Geometry: final body of the model. Coordinates: model frame, mm. Face numbers are marked on the shaded views. A direction names the side the tool comes from. Coordinates: 2 decimals unless noted, no trailing zeros. Loops run counter-clockwise (first coordinate to the right, second up) from the corner with the lowest first, then second, coordinate; pieces in that order, holes last. Notation, with made-up numbers: (17.25, 1) -> (63.25, 1) arc R15 ccw to (63.25, 6) -> close; hole circle Ø1 at (65.25, 55.25). An arc over 180 degrees is marked (long way). One line per item, written item: value. Start each with the question number.
Autodesk Inventor part; units mm, degrees
ref_plane "YZ Plane" through (0, 0, 0) normal (1, 0, 0) x (0, 1, 0)
ref_plane "XZ Plane" through (0, 0, 0) normal (0, 1, 0) x (-1, 0, 0)
ref_plane "XY Plane" through (0, 0, 0) normal (0, 0, 1) x (1, 0, 0)
sketch "Sketch1" plane through (0, 0, 0) normal (0, 1, 0) x (-1, 0, 0)
  line L0 (12.9507, 24.0308) -> (-67.0493, 24.0308)
  line L1 (-67.0493, 24.0308) -> (-67.0493, -25.9692)
  line L2 (-67.0493, -25.9692) -> (12.9507, -25.9692)
  line L3 (12.9507, -25.9692) -> (12.9507, 24.0308)
  point P0 (0, 0)
  dimension "d0" = 80
  dimension "d1" = 50
extrude "Extrusion1" add sketch "Sketch1" along normal blind 86
sketch "Sketch2" plane through (0, 0, 0) normal (0, -1, 0) x (1, 0, 0)
  circle A0 centre (27.0493, -0.9692) radius 20
  point P0 (0, 0)
  point P1 (67.0493, -25.9692)
  point P2 (-12.9507, 24.0308)
  dimension "d7" = 40
sketch "Sketch3" plane through (67.0493, 0, -25.9692) normal (0, 0, -1) x (-1, 0, 0)
  circle A0 centre (40, 43) radius 40
  circle A1 centre (40, 43) radius 25
  line L0 (0, 0) -> (15, 0)
  line L1 (0, 0) -> (80, 0)
  line L2 (80, 0) -> (65, 0)
  line L3 (65, 0) -> (65, 11.775)
  line L4 (15, 0) -> (15, 11.775)
  line L5 (0, 86) -> (80, 86)
  line L6 (0, 86) -> (80, 86)
  line L7 (80, 86) -> (80, 0)
  line L8 (80, 0) -> (0, 0)
  line L9 (0, 0) -> (0, 86)
  point P0 (67.0493, 0)
  point P1 (0, 43)
  point P2 (80, 43)
  dimension "d10" = 50
  dimension "d15" = 15
  dimension "d16" = 15
extrude "Extrusion2" cut sketch "Sketch3" against normal blind 100 contours A1
extrude "Extrusion3" cut sketch "Sketch2" against normal blind 47.6125
extrude "Extrusion4" cut sketch "Sketch3" against normal blind 100 contours L4 L0 L9 A0
extrude "Extrusion5" cut sketch "Sketch3" against normal blind 100 contours A0 L7 L1 L3
extrude "Extrusion6" cut sketch "Sketch3" against normal blind 100 contours L9 L5 L7 A0
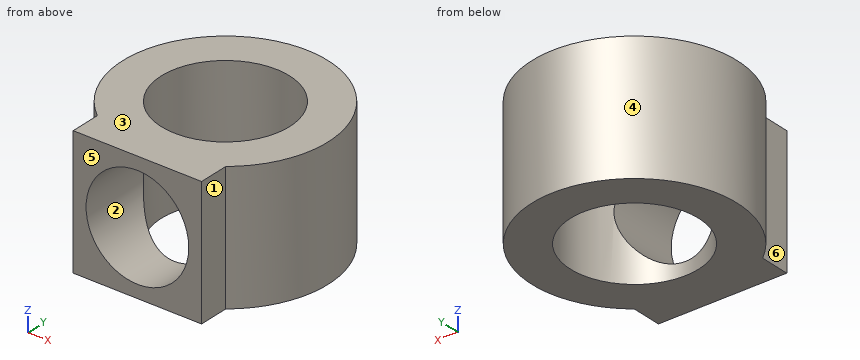
1. Section C-C on x = 48.5. Return the cut outline in (y, z).
2. Pin query (flat end, axial travel): pin 1 Ø3.5 at (y, z) = (8, 5.5) entering from +X; pin 2 Ø24 at (x, z) = (27.05, -0.97) entering from +Y; pin 3 Ø13 at (y, z) = (6, -13) entering from -X. Return the tip coordinate at first contact, or that it passes through.
3. Section A-A on y = 43. Return the cut outline in (x, z).
4. Section B-B on z = -22.5. Return the cut outline in (x, y) (3 decimals).
5. Draft query along X for the marked faces 1, 2, 3 and 4. Return one class per face: released by +X, released by -X, zero draft, split by the parting line, or undercut.
6. Set-up query: the marked faces 5 and 6. Return all of +Z, -Z, +X, -X, +Y, -Y with unobstructed straight access to the full face (end or side cutting, diameter ignored); none if empty.
7. Line query: L1, parallel to X at y = 5.5, z = -1.5; L2, parallel to X at y = 63, z = -20.5; L3, parallel to Y at x = 5.5, z = 12. Output: solid intervals per line, ascending. Write a range as [from, to].
8. Section D-D on x = 12. Return the cut outline in (y, z).
Checks:
1. outline: (0, -25.97) -> (30.16, -25.97) -> (30.16, 24.03) -> (0, 24.03) -> close; (55.84, -25.97) -> (76.76, -25.97) -> (76.76, 24.03) -> (55.84, 24.03) -> close
2. pin 1: x = 52.05
2. pin 2: y = 83
2. pin 3: x = 1.17
3. outline: (-12.95, -25.97) -> (2.05, -25.97) -> (2.05, 24.03) -> (-12.95, 24.03) -> close; (52.05, -25.97) -> (67.05, -25.97) -> (67.05, 24.03) -> (52.05, 24.03) -> close
4. outline: (2.049, 0) -> (52.049, 0) -> (52.049, 11.775) arc R40 ccw (long way) to (2.049, 11.775) -> close; hole circle Ø50 at (27.049, 43)
5. face 1: released by +X
5. face 2: undercut
5. face 3: zero draft
5. face 4: split by the parting line
6. face 5: +Z, -Z, +X, -X, -Y
6. face 6: +Z, -Z, -X, -Y
7. L1: [2.05, 7.06], [47.04, 52.05]
7. L2: [-7.59, 12.05], [42.05, 61.69]
7. L3: [0, 30.33], [55.67, 76.7]
8. outline: (0, -25.97) -> (23.04, -25.97) -> (23.04, -14.14) -> (0, -14.14) -> close; (0, 12.2) -> (23.04, 12.2) -> (23.04, 24.03) -> (0, 24.03) -> close; (62.96, -25.97) -> (80.06, -25.97) -> (80.06, 24.03) -> (62.96, 24.03) -> close
